Input: dimensioned drawing with shaded views. Units: mm. Origin: part minimum x, y, z. A direction names the side the tool comes from. Round coordinates to 2 decimals unless told otherwise and drop trailing zeros. Write each loop counter-clockwise with the first axis right and the second up, starting at its lowest first coordinate (ties: lowest second). Pieces come first, ordered by that corner, then holes. Notation, with made-up numbers: (25.25, 44.25) - (60.25, 44.25) arc R17 cw to (60.25, 77.25) - close; hole circle Ø4 at (22, 67.5). An arc over 180 degrees is marked (long way). Use one line per item in the form item = value.
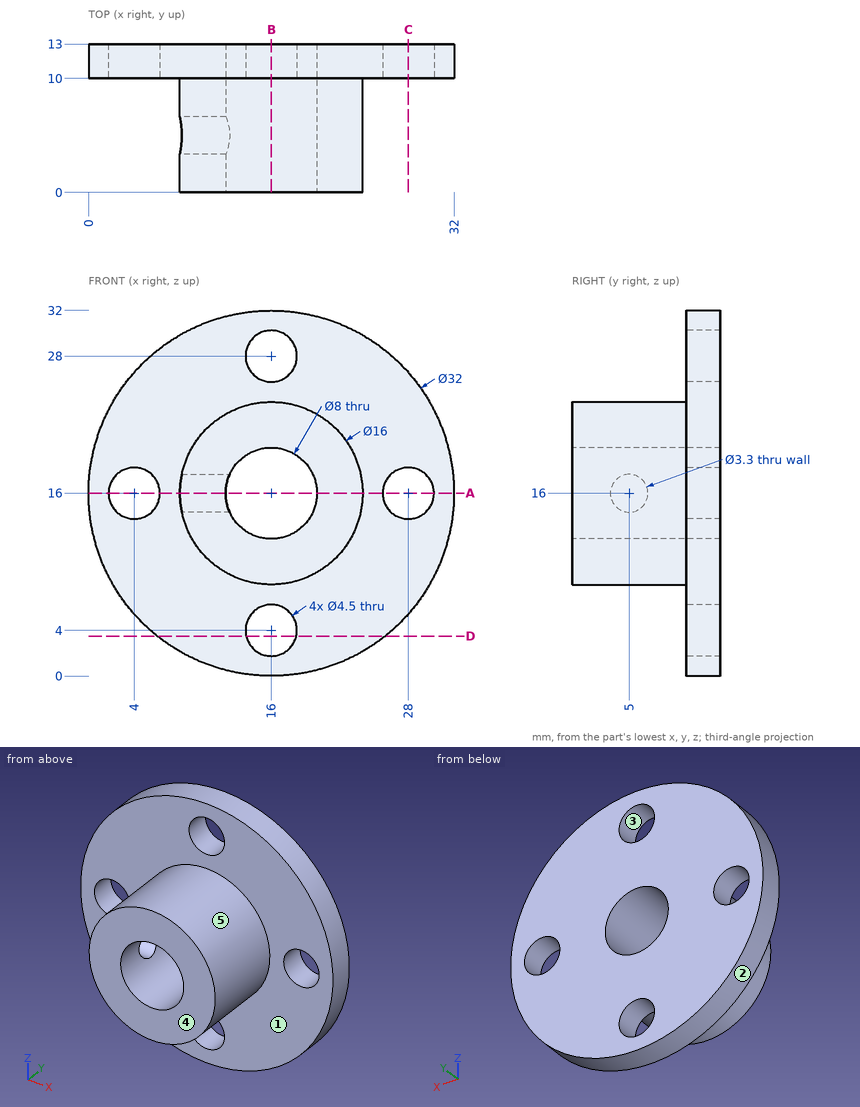
(1) Access query for the marked faces 1 and 2. Directions: +Z, -Z, +X, -X, +Y, -Y. A direction counts if a zero-diameter tool reaches every point of the face in a straight line with its end or side. Return the directions, or none.
Derived:
face_1 = -Y
face_2 = +Y, -Y
(2) Draft query along Z for the marked faces 3, 4 and 5. Return one class per face: released by +Z, released by -Z, zero draft, split by the parting line, or undercut.
Derived:
face_3 = undercut
face_4 = zero draft
face_5 = split by the parting line
(3) Cut plane C-C on x = 28. Output: boundary loops of the cut face in (y, z).
Derived:
outline = (10, 5.42) - (13, 5.42) - (13, 13.75) - (10, 13.75) - close; (10, 18.25) - (13, 18.25) - (13, 26.58) - (10, 26.58) - close
(4) Material intervals for L1, parallel to X at y = 11.1, z = 16; L2, parallel to X at y = 7.75, z = 16; L3, parallel to Y at x = 8.9, z = 16, sorted ascending.
Derived:
L1 = 0 to 1.75, 6.25 to 12, 20 to 25.75, 30.25 to 32
L2 = 8 to 12, 20 to 24
L3 = 0 to 3.35, 6.65 to 13
(5) Cut plane A-A on z = 16. Output: boundary loops of the cut face in (x, y), then the cut area to 3 significant figures.
Derived:
outline = (0, 10) - (1.75, 10) - (1.75, 13) - (0, 13) - close; (6.25, 10) - (8, 10) - (8, 6.65) - (12, 6.65) - (12, 13) - (6.25, 13) - close; (8, 0) - (12, 0) - (12, 3.35) - (8, 3.35) - close; (20, 0) - (24, 0) - (24, 10) - (25.75, 10) - (25.75, 13) - (20, 13) - close; (30.25, 10) - (32, 10) - (32, 13) - (30.25, 13) - close
area = 112 mm^2
(6) Cut plane D-D on z = 3.5. Output: boundary loops of the cut face in (x, y), then the cut area to 3 significant figures.
Derived:
outline = (6.01, 10) - (13.81, 10) - (13.81, 13) - (6.01, 13) - close; (18.19, 10) - (25.99, 10) - (25.99, 13) - (18.19, 13) - close
area = 46.8 mm^2
(7) Cut plane B-B on x = 16. Output: boundary loops of the cut face in (y, z).
Derived:
outline = (0, 8) - (10, 8) - (10, 6.25) - (13, 6.25) - (13, 12) - (0, 12) - close; (0, 20) - (13, 20) - (13, 25.75) - (10, 25.75) - (10, 24) - (0, 24) - close; (10, 0) - (13, 0) - (13, 1.75) - (10, 1.75) - close; (10, 30.25) - (13, 30.25) - (13, 32) - (10, 32) - close
(8) First-contact query: pin 1 Ø3.5 at (x, z) = (16, 28) entering from -Y; pin 2 Ø6 at (y, z) = (11, 21) entering from -X; pin 3 Ø6 at (y, z) = (3.5, 22.5) entering from -X; pin 4 Ø2 at (y, z) = (5, 16) entering from -X. Flat tips, straight axial feed; report the tip coordinate or a pass-through.
Derived:
pin_1 = through
pin_2 = 0.13
pin_3 = 8.81
pin_4 = 19.87
